Could you check a few things on this drawing? It's one solid part, dimensions in mm from its lowest x, y, z. A direction names the side the tool comes from. Coordinates: 2 decimals unless noted, no trailing zeros. Order: outer loops, then holes, each group sorted by start corner. A loop starts at its lowest first (then second) coordinate and runs counter-clockwise, first axis right, second up. Notation, with made-up numbers: (82.25, -38.75) - (137.25, -38.75) arc R23 cw to (137.25, -14.75) - close; hole circle Ø1 at (83.25, 47.5). An arc over 180 degrees is marked (long way). Return JSON: item names as keys, results as strings. Group by question number.
1) Imagine slicing it at B-B (z = 10.5). Write out the boundary of the cut face in (x, y), and give its area (3 significant figures).
2) If we mould it in two halves opening along X, with no side actions, what happens to the marked faces 1, 2 and 3? For each: pulls with the +X half, pulls with the -X half, needs draft (parallel to the pull), parting line crosses it, or undercut.
3) Which directions (+Z, -Z, +X, -X, +Y, -Y) give clear straight access to the entire face, cutting with the end or side of a thin tool? Please do the marked faces 4, 5, 6 and 7.
4) Imagine slicing it at A-A (x = 27.5). Write out the boundary of the cut face in (y, z), and give its area (3 significant figures).
5) Imagine slicing it at C-C (y = 1.3). Write out the boundary of the cut face in (x, z).
6) Imagine slicing it at D-D (z = 5.75). Write out the boundary of the cut face in (x, y), and give its area (3 significant figures).
7) If I drill on line 1 along X through (y, z) = (0.95, 10.5); line 2 along X through (y, z) = (4.7, 15.25); line 3 along Y through (x, z) = (27.5, 5.25), over which ranges is the centre line in solid material (lowest first)?
8) For pin 1 Ø2.5 at (x, z) = (29.5, 11.5) entering from +Y; pin 2 Ø2.5 at (x, y) = (29, 4) entering from +Z; pin 3 Ø4 at (x, z) = (37, 7) entering from -Y; pin 4 Ø2 at (x, y) = (41.5, 2) entering from -Z, each with a flat end and sliding along its axis, tell me the tip position at first contact or that it passes through.
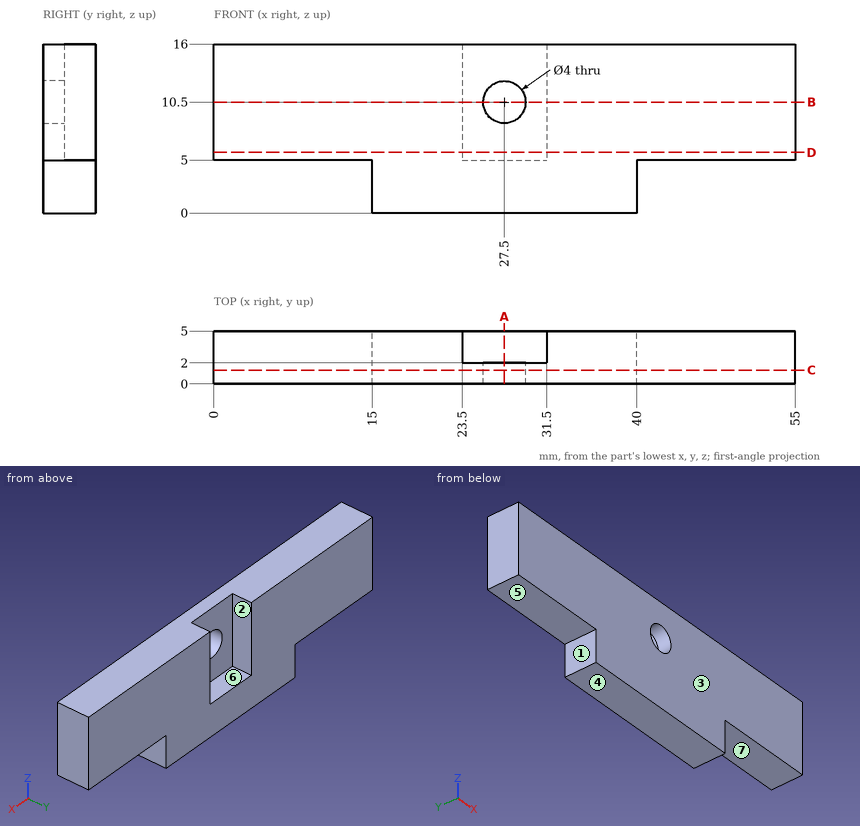
Calculated:
{
 "1": {"outline": "(0, 0) - (25.5, 0) - (25.5, 2) - (23.5, 2) - (23.5, 5) - (0, 5) - close; (29.5, 0) - (55, 0) - (55, 5) - (31.5, 5) - (31.5, 2) - (29.5, 2) - close", "area": "243 mm2"},
 "2": {"face 1": "pulls with the -X half", "face 2": "undercut", "face 3": "needs draft"},
 "3": {"face 4": "-Z, +X, -X, +Y, -Y", "face 5": "-Z, -X, +Y, -Y", "face 6": "+Z, +Y", "face 7": "-Z, +X, +Y, -Y"},
 "4": {"outline": "(0, 0) - (5, 0) - (5, 5) - (2, 5) - (2, 8.5) - (0, 8.5) - close; (0, 12.5) - (2, 12.5) - (2, 16) - (0, 16) - close", "area": "39.0 mm2"},
 "5": {"outline": "(0, 5) - (15, 5) - (15, 0) - (40, 0) - (40, 5) - (55, 5) - (55, 16) - (0, 16) - close; hole circle Ø4 at (27.5, 10.5)"},
 "6": {"outline": "(0, 0) - (55, 0) - (55, 5) - (31.5, 5) - (31.5, 2) - (23.5, 2) - (23.5, 5) - (0, 5) - close", "area": "251 mm2"},
 "7": {"line 1": "0 to 25.5, 29.5 to 55", "line 2": "0 to 23.5, 31.5 to 55", "line 3": "0 to 2"},
 "8": {"pin 1": "y = 2", "pin 2": "z = 5", "pin 3": "y = 0", "pin 4": "z = 5"}
}
